The listing builds one solid part. Answer for the finished solid, in the listing's coordinates (mm). A direction names the side the tool comes from. Coordinates: 2 decimals unless noted, no trailing zeros. Order: outer loops, then holes, each group sorted by start corner. A loop starts at its lowest first (then second) coordinate and runs counter-clockwise, first axis right, second up. Notation, with made-up numbers: (24.25, -37.75) -> (55.25, -37.75) arc R23 ccw to (55.25, -0.75) -> close; hole circle Ø9 at (-31.5, 41). An arc over 180 degrees is marked (long way). Return JSON: item names as keys, results as strings.
```python
from build123d import *

# Parameters (mm, degrees)
SKETCH2_R           = 3.5
BOSS_EXTRUDE1_DEPTH = 3.65
SKETCH3_R           = 2.675
BOSS_EXTRUDE2_DEPTH = 1.95
SKETCH4_R           = 3.575
BOSS_EXTRUDE3_DEPTH = 22.4
SKETCH5_R           = 2.675
BOSS_EXTRUDE4_DEPTH = 1.95
SKETCH6_R           = 3.5
BOSS_EXTRUDE5_DEPTH = 3.65


with BuildPart() as part:
    # Sketch2 → Boss-Extrude1 (new body)
    with BuildSketch(Plane(origin=(0, 0, 0), x_dir=(1, 0, 0), z_dir=(0, 1, 0))):
        Circle(SKETCH2_R)
    extrude(amount=BOSS_EXTRUDE1_DEPTH)

    # Sketch3 → Boss-Extrude2 (add)
    with BuildSketch(Plane(origin=(0, 3.65, 0), x_dir=(1, 0, 0), z_dir=(0, 1, 0))):
        Circle(SKETCH3_R)
    extrude(amount=BOSS_EXTRUDE2_DEPTH)

    # Sketch4 → Boss-Extrude3 (add)
    with BuildSketch(Plane(origin=(0, 5.6, 0), x_dir=(1, 0, 0), z_dir=(0, 1, 0))):
        Circle(SKETCH4_R)
    extrude(amount=BOSS_EXTRUDE3_DEPTH)

    # Sketch5 → Boss-Extrude4 (add)
    with BuildSketch(Plane(origin=(0, 28, 0), x_dir=(1, 0, 0), z_dir=(0, 1, 0))):
        Circle(SKETCH5_R)
    extrude(amount=BOSS_EXTRUDE4_DEPTH)

    # Sketch6 → Boss-Extrude5 (add)
    with BuildSketch(Plane(origin=(0, 29.95, 0), x_dir=(1, 0, 0), z_dir=(0, 1, 0))):
        Circle(SKETCH6_R)
    extrude(amount=BOSS_EXTRUDE5_DEPTH)


solid = part.part
```
Item 1: The part is cut by section C-C on y = 29. Determine the outline of the cut face in (x, z) (3 decimals), plus the area to 3 significant figures.
Answer list:
{"outline": "circle Ø5.35 at (0, 0)", "area": "22.5 mm2"}
Item 2: The part is cut by section A-A on z = 0. Determine the outline of the cut face in (x, y) (3 decimals).
Answer list:
{"outline": "(-3.575, 5.6) -> (-2.675, 5.6) -> (-2.675, 3.65) -> (-3.5, 3.65) -> (-3.5, 0) -> (3.5, 0) -> (3.5, 3.65) -> (2.675, 3.65) -> (2.675, 5.6) -> (3.575, 5.6) -> (3.575, 28) -> (2.675, 28) -> (2.675, 29.95) -> (3.5, 29.95) -> (3.5, 33.6) -> (-3.5, 33.6) -> (-3.5, 29.95) -> (-2.675, 29.95) -> (-2.675, 28) -> (-3.575, 28) -> close"}
Item 3: Find the intervals of material crossed by probe 1 along Y at (x, z) = (2.75, 1); probe 2 along X at (y, z) = (15, 3.25); probe 3 along X at (y, z) = (25, 3), in increasing order.
Answer list:
{"probe 1": "0 to 3.65, 5.6 to 28, 29.95 to 33.6", "probe 2": "-1.49 to 1.49", "probe 3": "-1.94 to 1.94"}
Item 4: The part is cut by section B-B on x = 0. Determine the outline of the cut face in (y, z) (3 decimals).
Answer list:
{"outline": "(0, -3.5) -> (3.65, -3.5) -> (3.65, -2.675) -> (5.6, -2.675) -> (5.6, -3.575) -> (28, -3.575) -> (28, -2.675) -> (29.95, -2.675) -> (29.95, -3.5) -> (33.6, -3.5) -> (33.6, 3.5) -> (29.95, 3.5) -> (29.95, 2.675) -> (28, 2.675) -> (28, 3.575) -> (5.6, 3.575) -> (5.6, 2.675) -> (3.65, 2.675) -> (3.65, 3.5) -> (0, 3.5) -> close"}
Item 5: Determine the mould class of faces 4 (the flat face through (-1, 29.95, 3)), 5 (the flat face through (0, 33.6, 0)), 6 (the cylindrical face through (3.233, 1.799, 1.341)), 7 (the flat face through (0, 0, 0)) for opening direction Y: pulls with the +Y half, pulls with the -Y half, needs draft (parallel to the pull), parting line crosses it, or undercut.
Answer list:
{"face 4": "undercut", "face 5": "pulls with the +Y half", "face 6": "needs draft", "face 7": "pulls with the -Y half"}
Item 6: Flat-ended cylindrical pins translate along their axes: pin 1 (3 mm diameter, centred on x = 2, y = 14, fed in from -Z); pin 2 (1 mm diameter, centred on x = -2.5, y = 6.5, fed in from +Z). Find the tip coordinate at first contact, or state that the pin passes through.
Answer list:
{"pin 1": "z = -3.54", "pin 2": "z = 2.96"}
Item 7: Which of the six approach directions +Z, -Z, +X, -X, +Y, -Y give full straight-line access (tool end or side, diameter ignored) to faces 1 (the cylindrical face through (-0.465, 16.643, -3.545)), 2 (the cylindrical face through (-0.58, 28.96, 2.61)), 3 (the cylindrical face through (3.233, 31.749, 1.341))?
Answer list:
{"face 1": "+Y, -Y", "face 2": "none", "face 3": "+Y"}
